from build123d import *

# Parameters (mm, degrees)
SKETCH1_W               = 152.4
SKETCH1_H               = 251.46
BOSS_EXTRUDE1_DEPTH     = 6.35
SKETCH2_W               = 19.05
SKETCH2_H               = 6.35
SKETCH2_W_2             = 12.7
CUT_EXTRUDE1_DEPTH      = 6.35
SKETCH3_W               = 19.05
SKETCH3_H               = 6.35
SKETCH3_W_2             = 12.7
CUT_EXTRUDE2_DEPTH      = 1
CUT_EXTRUDE2_DEPTH_BACK = 6.35
SKETCH4_W               = 6.35
SKETCH4_H               = 25.4
SKETCH4_H_2             = 43.18
CUT_EXTRUDE3_DEPTH      = 6.35
SKETCH5_R               = 44.45
CUT_EXTRUDE4_DEPTH      = 7.35
SKETCH6_W               = 117.22
SKETCH6_H               = 65.22
SKETCH6_R               = 1.75
CUT_EXTRUDE5_DEPTH      = 7.35


with BuildPart() as part:
    # Sketch1 → Boss-Extrude1 (new body)
    with BuildSketch(Plane.XY):
        with Locations((-209.55, -120.65)):
            Rectangle(SKETCH1_W, SKETCH1_H)
    extrude(amount=BOSS_EXTRUDE1_DEPTH)

    # Sketch2 → Cut-Extrude1 (cut)
    with BuildSketch(Plane(origin=(0, 5.08, 0), x_dir=(1, 0, 0), z_dir=(0, 1, 0))):
        with Locations((-250.825, -3.175)):
            Rectangle(SKETCH2_W, SKETCH2_H)
        with Locations((-206.375, -3.175)):
            Rectangle(SKETCH2_W, SKETCH2_H)
        with Locations((-165.1, -3.175)):
            Rectangle(SKETCH2_W_2, SKETCH2_H)
    extrude(amount=-CUT_EXTRUDE1_DEPTH, mode=Mode.SUBTRACT)

    # Sketch3 → Cut-Extrude2 (cut, two sides)
    with BuildSketch(Plane.XZ.offset(246.38)) as cut_extrude2_sk:
        with Locations((-250.825, 3.175)):
            Rectangle(SKETCH3_W, SKETCH3_H)
        with Locations((-206.375, 3.175)):
            Rectangle(SKETCH3_W, SKETCH3_H)
        with Locations((-165.1, 3.175)):
            Rectangle(SKETCH3_W_2, SKETCH3_H)
    extrude(amount=CUT_EXTRUDE2_DEPTH, mode=Mode.SUBTRACT)
    extrude(cut_extrude2_sk.sketch, amount=-CUT_EXTRUDE2_DEPTH_BACK, mode=Mode.SUBTRACT)

    # Sketch4 → Cut-Extrude3 (cut)
    with BuildSketch(Plane.XY.offset(6.35)):
        with Locations((-136.525, -152.4)):
            Rectangle(SKETCH4_W, SKETCH4_H)
        with Locations((-136.525, -101.6)):
            Rectangle(SKETCH4_W, SKETCH4_H)
        with Locations((-136.525, -16.51)):
            Rectangle(SKETCH4_W, SKETCH4_H_2)
        with Locations((-136.525, -228.6)):
            Rectangle(SKETCH4_W, SKETCH4_H)
    extrude(amount=-CUT_EXTRUDE3_DEPTH, mode=Mode.SUBTRACT)

    # Sketch5 → Cut-Extrude4 (cut, through all)
    with BuildSketch(Plane.XY.offset(6.35)):
        with Locations((-321.31, -120.65)):
            Circle(SKETCH5_R)
    extrude(amount=-CUT_EXTRUDE4_DEPTH, mode=Mode.SUBTRACT)

    # Sketch6 → Cut-Extrude5 (cut, through all)
    with BuildSketch(Plane.XY.offset(6.35)):
        with Locations((-211.01, -124.87)):
            Rectangle(SKETCH6_W, SKETCH6_H)
        with Locations((-273.51, -88.37)):
            Circle(SKETCH6_R)
        with Locations((-273.51, -161.37)):
            Circle(SKETCH6_R)
        with Locations((-148.51, -88.37)):
            Circle(SKETCH6_R)
        with Locations((-148.51, -161.37)):
            Circle(SKETCH6_R)
    extrude(amount=-CUT_EXTRUDE5_DEPTH, mode=Mode.SUBTRACT)


solid = part.part
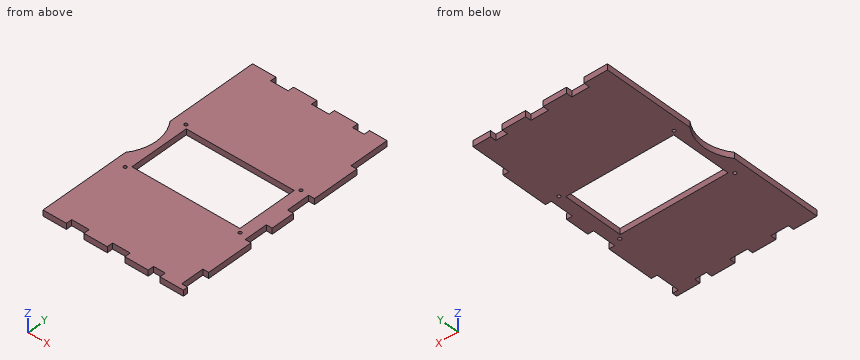
Build history of the part. All positions in model axes, mm. Give positions to 0.01 mm unless a question says otherwise; leave off trailing zeros. Loops run counter-clockwise (first coordinate to the right, second up) from the corner with the lowest first, then second, coordinate; pieces in that order, holes last. Notation, with made-up numbers: (5.25, 53) - (20.25, 53) arc R28 cw to (20.25, 78) - close; hole circle Ø9 at (47.25, 9.5). An arc over 180 degrees is marked (long way). Write item = value, one per line. Start each with the question number.
1) Drop flat-ended pins along their axis: pin 1 Ø3 at (y, z) = (-23.5, 4) entering from +X; pin 2 Ø1.9 at (x, z) = (-167, 4) entering from -Y. Give the stop position or say it passes through.
2) Band-saw the part on A-A on x = -201.5. Give the cut face in (y, z).
3) Band-saw the part on B-B on z = 4. Count the separate pieces of the cut face and the enclosed holes in it, plus the area to 3 significant figures.
4) Probe probe 1 along Y at (x, z) = (-148.51, 4); probe 2 along X at (y, z) = (-161.37, 2); probe 3 along X at (y, z) = (-88.37, 3). List the from-to ranges inside material, lowest first. Write a range as from..to.
Final values:
q1.pin_1 = -139.7
q1.pin_2 = -240.03
q2.outline = (-240.03, 0) - (-157.48, 0) - (-157.48, 6.35) - (-240.03, 6.35) - close; (-92.26, 0) - (-1.27, 0) - (-1.27, 6.35) - (-92.26, 6.35) - close
q3.separate_pieces = 1
q3.enclosed_holes = 5
q3.area = 28,900 mm²
q4.probe_1 = -246.38..-163.12, -159.62..-90.12, -86.62..5.08
q4.probe_2 = -285.75..-275.26, -271.76..-150.26, -146.76..-139.7
q4.probe_3 = -285.75..-275.26, -271.76..-150.26, -146.76..-133.35
